Model file for the job. Use its own axes, mm. A direction names the side the tool comes from. Round coordinates to 2 decimals unless told otherwise and drop trailing zeros. Write each loop counter-clockwise with the first axis right and the second up, starting at its lowest first coordinate (ties: lowest second). Pieces come first, ordered by that corner, then holes.
Autodesk Inventor part; units mm, degrees
ref_plane "YZ Plane" through (0, 0, 0) normal (1, 0, 0) x (0, 1, 0)
ref_plane "XZ Plane" through (0, 0, 0) normal (0, 1, 0) x (-1, 0, 0)
ref_plane "XY Plane" through (0, 0, 0) normal (0, 0, 1) x (1, 0, 0)
sketch "スケッチ1" plane through (0, 0, 0) normal (0, 1, 0) x (-1, 0, 0)
  line L0 (0, 0) -> (20, 0)
  line L1 (20, 0) -> (20, -20)
  line L2 (20, -20) -> (0, -20)
  line L3 (0, -20) -> (0, 0)
  line L4 (17.5, -2.5) -> (2.5, -2.5)
  line L5 (2.5, -2.5) -> (2.5, -17.5)
  line L6 (2.5, -17.5) -> (17.5, -17.5)
  line L7 (17.5, -17.5) -> (17.5, -2.5)
  dimension "d0" = 20
  dimension "d1" = 20
  dimension "d2" = 15
  dimension "d3" = 15
  dimension "d4" = 2.5
  dimension "d5" = 2.5
extrude "押し出し1" add sketch "スケッチ1" along normal blind 15
sketch "スケッチ2" plane through (-20, 0, 0) normal (0, 0, 1) x (1, 0, 0)
  line L0 (20, 0) -> (-55, 0)
  line L1 (-55, 0) -> (-55, 17.5)
  line L2 (-55, 17.5) -> (20, 17.5)
  line L3 (20, 17.5) -> (20, 0)
  line L4 (-55, 17.5) -> (-45, 17.5)
  line L5 (-45, 17.5) -> (-45, 14.5)
  line L6 (-45, 14.5) -> (-55, 14.5)
  line L7 (-55, 14.5) -> (-55, 17.5)
  line L8 (0, 0) -> (0, 15)
  line L9 (-55, 14.5) -> (0, 0)
  line L10 (-45, 17.5) -> (0, 15)
  point P0 (-45, 17.5)
  dimension "d8" = 75
  dimension "d9" = 17.5
  dimension "d10" = 10
  dimension "d11" = 3
extrude "押し出し2" add sketch "スケッチ2" against normal blind 20 contours L9 L6 L5 L10 L8 | L1 L2 L5 L6
sketch "スケッチ3" plane through (0, 0, 0) normal (0, -1, 0) x (1, 0, 0)
  line L0 (-75, 0) -> (-75, -20)
  line L1 (0, 0) -> (0, -20)
  line L2 (-75, -14) -> (0, -14)
  line L3 (0, -14) -> (0, -6)
  line L4 (0, -6) -> (-75, -6)
  line L5 (-75, -6) -> (-75, -14)
  line L6 (-20, -20) -> (-75, -20)
  line L7 (-75, -14) -> (-20, -20)
  line L8 (-20, 0) -> (0, 0)
  line L9 (-75, -6) -> (-20, 0)
  line L10 (-75, -20) -> (-20, -20)
  line L11 (-20, -20) -> (-20, 0)
  line L12 (-20, 0) -> (-75, 0)
  line L13 (-75, 0) -> (-75, -20)
  dimension "d14" = 8
  dimension "d15" = 6
extrude "押し出し3" cut sketch "スケッチ3" against normal through all contours L12 L9 L0 | L7 L6 L0
sketch "スケッチ4" plane through (0, 0, 0) normal (1, 0, 0) x (0, 0, -1)
  line L0 (0, 0) -> (0, 15)
  line L1 (0, 7.5) -> (20, 7.5)
  line L2 (20, 0) -> (20, 15)
  point P0 (10, 7.5)
hole "穴1" at (0, 7.5, -10) direction (-1, 0, 0) diameter 3.2 depth 8 tip angle 118
properties part number "endeff_3dp4" material "ABS プラスチック"
1) Pull direction X, two halves, no side cores. Call faces 1 (the face through (-10, 7, -17.5)), 2 (the face through (-10, 15, -19)), 3 (the face through (-41.774, 10.572, -17.625)): released by +X, released by -X, zero draft, split by the parting line, or undercut.
2) Which spindle directions (+Z, -Z, +X, -X, +Y, -Y) get a long thin tool onto all of the face, cutting with end or side? Do faces 4 (the face through (-10, 0, -19)), 5 (the face through (-1.27, 8.47, -8.73)), 6 (the face through (-17.5, 7, -10)). Say none if no direction does.
3) Cut at B-B on x = -6. List the corners of the cut face in (y, z).
4) Cut at A-A on z = -6.75. List the corners of the cut face in (x, y), and give its area (4 significant figures).
5) Flat gauge pins, fed straight in: pin 1 Ø10 at (y, z) = (7.5, -15) entering from +X; pin 2 Ø1.5 at (x, z) = (-24, -13.5) entering from +Y; pin 3 Ø5 at (x, y) = (-51, 11.5) entering from -Z; pin 4 Ø6 at (x, z) = (-58.5, -12.5) entering from +Y. Where does each tip first touch, or does it go through?
6) Cut at D-D on y = 3.5. List the corners of the cut face in (x, z).
7) Wall check: probe 1 along Y at (x, z) = (-0.55, -10); probe 2 along Z at (x, y) = (-0.65, 7.5); probe 3 along Z at (x, y) = (-7.5, 9). Give the ranges that are in metal, low to high.
8) Cut at C-C on z = -10. List the corners of the cut face in (x, y).
Result sheet:
1. face 1: undercut
1. face 2: zero draft
1. face 3: released by -X
2. face 4: +Z, -Z, +X, -X, -Y
2. face 5: +X
2. face 6: +Y, -Y
3. outline: (0, -20) - (15, -20) - (15, -17.5) - (0, -17.5) - close; (0, -2.5) - (15, -2.5) - (15, 0) - (0, 0) - close
4. outline: (-75, 14.5) - (-20, 0) - (-17.5, 0) - (-17.5, 15) - (-20, 15) - (-65, 17.5) - (-75, 17.5) - close; (-2.5, 0) - (0, 0) - (0, 15) - (-2.5, 15) - close
4. area: 582.5 mm2
5. pin 1: stops at x = 0
5. pin 2: stops at y = 15.26
5. pin 3: stops at z = -16.89
5. pin 4: stops at y = 17.31
6. outline: (-33.28, -18.55) - (-20, -20) - (0, -20) - (0, 0) - (-20, 0) - (-33.28, -1.45) - close; hole (-17.5, -17.5) - (-2.5, -17.5) - (-2.5, -2.5) - (-17.5, -2.5) - close
7. probe 1: y = 0 to 5.9, 9.1 to 15
7. probe 2: z = -20 to -11.6, -8.4 to 0
7. probe 3: z = -20 to -17.5, -2.5 to 0
8. outline: (-75, 14.5) - (-20, 0) - (-17.5, 0) - (-17.5, 15) - (-20, 15) - (-65, 17.5) - (-75, 17.5) - close; (-2.5, 0) - (0, 0) - (0, 5.9) - (-2.5, 5.9) - close; (-2.5, 9.1) - (0, 9.1) - (0, 15) - (-2.5, 15) - close
